Could you check a few things on this model? Use its own coordinates, in mm. Face numbers are marked on the shaded views. A direction names the side the tool comes from. Coordinates: 2 decimals unless noted, no trailing zeros. Order: outer loops, then holes, each group sorted by start corner. A loop starts at its lowest first (then second) coordinate and runs counter-clockwise, first axis right, second up. Notation, with made-up numbers: (30, 50) - (68, 50) arc R16 ccw to (68, 69) - close; hole circle Ø1 at (0, -23). An arc over 180 degrees is marked (long way). Answer as a JSON object with one key per item and string values. Group by question number.
(1) We'd pull the mould along Y, two halves only. Please class the marked faces 4, 5 and 6: pulls with the +Y half, pulls with the -Y half, needs draft (parallel to the pull), parting line crosses it, or undercut.
(2) Imagine slicing it at C-C, the plane y = 71. Write out the boundary of the cut face in (x, z).
(3) Will these pins go through, and if not, where does the flat tip stop? P1, Ø2.5, axis at y = 47.5, z = 1.5, coming from the +X side; P2, Ø3.5, axis at y = 60, z = 2.5, coming from the -X side; P3, Ø1.5, axis at x = -12.5, z = 1.5, coming from the -Y side.
(4) Imagine slicing it at B-B, the plane z = 7.25. Give the number of separate pieces and of enclosed holes in the cut face, and give its area (3 significant figures).
(5) Please list where these lines run through material, in increasing order: probe 1 along Y at (x, z) = (4, 1.75); probe 2 along Y at (x, z) = (0.5, 4.25); probe 3 along X at (y, z) = (133.5, 5.5).
(6) Which directions (+Z, -Z, +X, -X, +Y, -Y) give clear straight access to the entire face, cutting with the end or side of a thin tool? Please do the marked faces 1, 2 and 3.
(7) Imagine slicing it at A-A, the plane y = 3. Write out the boundary of the cut face in (x, z), and give its area (3 significant figures).
from build123d import *

# Parameters (mm, degrees)
SKETCH_R     = 6.5
SKETCH_R_2   = 2.5
SKETCH_R_3   = 1.5
PAD_DEPTH    = 10
FILLET_R     = 2.5
POCKET_DEPTH = 5


with BuildPart() as part:
    # Sketch → Pad (new body)
    with BuildSketch(Plane.XY):
        with BuildLine():
            ThreePointArc((-8.660254, -5), (5, -8.660254), (8.660254, 5))
            Line((8.660254, 5), (0, 20))
            Line((0, 150), (0, 20))
            Line((0, 150), (8.660254, 165))
            ThreePointArc((8.660254, 165), (7.138618, 177.002866), (-4.832824, 178.754645))
            Line((-4.832824, 178.754645), (-22.414778, 169.048885))
            ThreePointArc((-22.414778, 169.048885), (-24.304296, 167.213013), (-24.998366, 164.671563))
            Line((-24.998366, 164.671563), (-24.998366, 107.671563))
            ThreePointArc((-24.998366, 107.671563), (-23.534478, 104.136606), (-20, 102.671563))
            Line((-20, 17.320508), (-20, 102.671563))
            ThreePointArc((-20, 17.320508), (-19.659258, 14.732318), (-18.660254, 12.320508))
            Line((-8.660254, -5), (-18.660254, 12.320508))
        make_face()
        Circle(SKETCH_R, mode=Mode.SUBTRACT)
        with Locations((0, 170)):
            Circle(SKETCH_R_2, mode=Mode.SUBTRACT)
        with Locations((-3.5, 78.364)):
            Circle(SKETCH_R_3, mode=Mode.SUBTRACT)
        with Locations((-3.5, 59.364)):
            Circle(SKETCH_R_3, mode=Mode.SUBTRACT)
        with Locations((-10, 47.874)):
            Circle(SKETCH_R_3, mode=Mode.SUBTRACT)
        with BuildLine():
            ThreePointArc((-21.998366, 107.671563), (-19.998366, 105.671563), (-17.998366, 107.671563))
            Line((-17.998366, 107.671563), (-17.998366, 119.671563))
            ThreePointArc((-17.998366, 119.671563), (-19.998366, 121.671563), (-21.998366, 119.671563))
            Line((-21.998366, 119.671563), (-21.998366, 107.671563))
        make_face(mode=Mode.SUBTRACT)
        with BuildLine():
            ThreePointArc((-17.998366, 164.671563), (-19.998366, 166.671563), (-21.998366, 164.671563))
            Line((-21.998366, 164.671563), (-21.998366, 152.671563))
            ThreePointArc((-21.998366, 152.671563), (-19.998366, 150.671563), (-17.998366, 152.671563))
            Line((-17.998366, 152.671563), (-17.998366, 164.671563))
        make_face(mode=Mode.SUBTRACT)
        with BuildLine():
            ThreePointArc((-17.998366, 142.171563), (-19.998366, 144.171563), (-21.998366, 142.171563))
            Line((-21.998366, 142.171563), (-21.998366, 130.171563))
            ThreePointArc((-21.998366, 130.171563), (-19.998366, 128.171563), (-17.998366, 130.171563))
            Line((-17.998366, 130.171563), (-17.998366, 142.171563))
        make_face(mode=Mode.SUBTRACT)
    extrude(amount=PAD_DEPTH)

    # Fillet
    fillet_edges = [part.edges().sort_by_distance(p)[0] for p in [
        (-20, 102.671563, 5),
    ]]
    fillet(fillet_edges, radius=FILLET_R)

    # Sketch001 (on Face2 of Fillet) → Pocket (cut)
    with BuildSketch(Plane(origin=(0, 0, 0), x_dir=(1, 0, 0), z_dir=(0, 0, -1))):
        Polygon((-3.5, -81.539426), (-0.75, -79.951713), (-0.75, -76.776287), (-3.5, -75.188574), (-6.25, -76.776287), (-6.25, -79.951713), align=None)
        Polygon((-3.5, -62.539426), (-0.75, -60.951713), (-0.75, -57.776287), (-3.5, -56.188574), (-6.25, -57.776287), (-6.25, -60.951713), align=None)
        Polygon((-10, -51.049426), (-7.25, -49.461713), (-7.25, -46.286287), (-10, -44.698574), (-12.75, -46.286287), (-12.75, -49.461713), align=None)
    extrude(amount=-POCKET_DEPTH, mode=Mode.SUBTRACT)


solid = part.part
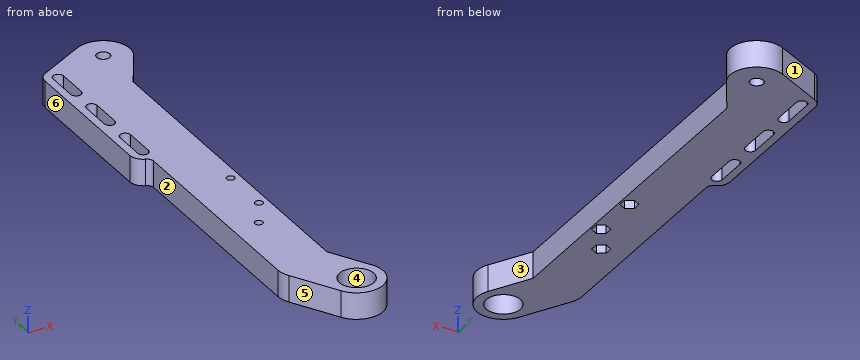
Result set:
{
 "1": {"face 4": "undercut", "face 5": "pulls with the -Y half", "face 6": "needs draft"},
 "2": {"outline": "(-20, 0) - (0, 0) - (0, 10) - (-20, 10) - close"},
 "3": {"P1": "stops at x = 0", "P2": "stops at x = -20", "P3": "stops at y = 0.35"},
 "4": {"separate pieces": "1", "enclosed holes": "8", "area": "3,890 mm^2"},
 "5": {"probe 1": "y = -9.17 to -5.12, 5.12 to 13.07, 156.93 to 179.17", "probe 2": "y = -9.99 to -6.48, 6.48 to 19.13, 150.87 to 167.55, 172.45 to 179.99", "probe 3": "x = -25 to -22, -18 to 0"},
 "6": {"face 1": "+Z, -Z, -X, +Y", "face 2": "+Z, -Z, -X, -Y", "face 3": "+Z, -Z, +X"},
 "7": {"outline": "(-13.28, 0) - (-5.77, 0) - (-5.77, 10) - (-13.28, 10) - close; (5.77, 0) - (9.54, 0) - (9.54, 10) - (5.77, 10) - close", "area": "113 mm^2"}
}
